```python
from build123d import *

# Parameters (mm, degrees)
F0_W           = 11
F0_H           = 30
F1_DEPTH       = 25
F1_DEPTH_BACK  = 25
F3_DEPTH       = 11
F4_R           = 10
F5_R           = 5
F6_DEPTH       = 12
F8_D           = 5
F8_START       = 11.4196012
F8_CSINK_D     = 10
F8_CSINK_ANGLE = 90


with BuildPart() as f1:
    # F0 (on Right) → F1 (new body, two sides)
    with BuildSketch(Plane.YZ) as f1_sk:
        with BuildLine():
            Line((-27.9105714739, 11), (-53.5, 11))
            Line((-53.5, 11), (-53.5, 0))
            Line((-53.5, 0), (-30, 0))
            ThreePointArc((-30, 0), (-29.4730143031, 5.5983415304), (-27.9105714739, 11))
        make_face()
        with BuildLine():
            ThreePointArc((27.9105714739, 11), (0, 30), (-27.9105714739, 11))
            ThreePointArc((-27.9105714739, 11), (-29.4730143031, 5.5983415304), (-30, 0))
            Line((-30, 0), (-19, 0))
            ThreePointArc((-19, 0), (0, 19), (19, 0))
            Line((19, 0), (30, 0))
            ThreePointArc((30, 0), (29.4730143031, 5.5983415304), (27.9105714739, 11))
        make_face()
        with BuildLine():
            Line((40, 11), (27.9105714739, 11))
            ThreePointArc((27.9105714739, 11), (29.4730143031, 5.5983415304), (30, 0))
            Line((30, 0), (51, 0))
            Line((51, 0), (51, 11))
            Line((51, 11), (40, 11))
        make_face()
        with Locations((45.5, 26)):
            Rectangle(F0_W, F0_H)
    extrude(amount=F1_DEPTH)
    extrude(f1_sk.sketch, amount=-F1_DEPTH_BACK)

    # F2 (on face) → F3 (cut)
    with BuildSketch(Plane(origin=(0, 51, 0), x_dir=(-1, 0, 0), z_dir=(0, 1, 0))):
        with BuildLine():
            Line((5, 41), (-5, 41))
            Line((-5, 41), (-5, 28.2676104225))
            ThreePointArc((-5, 28.2676104225), (0, 33.2676104225), (5, 28.2676104225))
            Line((5, 28.2676104225), (5, 41))
        make_face()
        with BuildLine():
            ThreePointArc((5, 28.2676104225), (0, 33.2676104225), (-5, 28.2676104225))
            Line((-5, 28.2676104225), (5, 28.2676104225))
        make_face()
        with BuildLine():
            Line((5, 28.2676104225), (-5, 28.2676104225))
            ThreePointArc((-5, 28.2676104225), (0, 23.2676104225), (5, 28.2676104225))
        make_face()
    extrude(amount=-F3_DEPTH, mode=Mode.SUBTRACT)

    # F4
    f4_edges = [f1.edges().sort_by_distance(p)[0] for p in [
        (25, -53.5, 5.5),
        (-25, -53.5, 5.5),
        (25, 45.5, 41),
        (-25, 45.5, 41),
    ]]
    fillet(f4_edges, radius=F4_R)

    # F5 (on face) → F6 (cut)
    with BuildSketch(Plane(origin=(0, 0, 0), x_dir=(1, 0, 0), z_dir=(0, 0, -1))):
        with Locations((-12, 43.5)):
            Circle(F5_R)
        with Locations((12, 43.5)):
            Circle(F5_R)
    extrude(amount=-F6_DEPTH, mode=Mode.SUBTRACT)

    # F8 (through all)
    # its depths count from where the whole tool has entered the part; down to there all is cleared
    with Locations(Plane.XY.offset(41).offset(-F8_START)):
        with Locations((0, 0)):
            CounterSinkHole(F8_D / 2, F8_CSINK_D / 2, counter_sink_angle=F8_CSINK_ANGLE)


solid = f1.part
```
Model file for the job. Use its own axes, mm. A direction names the side the tool comes from. Coordinates: 2 decimals unless noted, no trailing zeros. Write each loop counter-clockwise with the first axis right and the second up, starting at its lowest first coordinate (ties: lowest second). Pieces come first, ordered by that corner, then holes. Notation, with made-up numbers: (45, 31) - (95, 31) arc R30 ccw to (95, 65) - close; hole circle Ø7 at (44.25, 20.25). An arc over 180 degrees is marked (long way). Use a Markdown table: item, result. Add a question column.
Item 1: Drop flat-ended pins along their axis: pin 1 (1 mm diameter, centred on x = -19.5, z = 7, fed in from -Y); pin 2 (3 mm diameter, centred on x = -12.5, y = 5.5, fed in from +Z); pin 3 (5.5 mm diameter, centred on y = 48, z = 37, fed in from -X); pin 4 (9.5 mm diameter, centred on x = -5, y = 37, fed in from +Z). Give the stop position or say it passes through.
Item 2: Band-saw the part on B-B, the plane x = 12. Write the cut outline in (y, z), and give its area (3 significant figures).
Item 3: Two-plate mould, pull along X, no slides. Class faces 4 (the face through (0, -53.5, 6)), 5 (the face through (21.99, -50.65, 5.42)), 6 (the face through (-5, 0.11, 29.75)): pulls with the +X half, pulls with the -X half, needs draft (parallel to the pull), parting line crosses it, or undercut.
Item 4: Band-saw the part on D-D, the plane y = -37. Write the cut outline in (x, z).
Item 5: 3-axis set-ups, long thin cutter, end or side, ignore diameter. For faces 1 (the face through (0, 34, 11)), 2 (the face through (0, -41, 11)), 3 (the face through (5, -0.11, 29.75)): which of +Z, -Z, +X, -X, +Y, -Y reach the whole face in a straight line?
Item 6: Band-saw the part on A-A, the plane z = 7. Write the cut outline in (x, y).
Item 7: Drill centre lines: line 1 along X through (y, z) = (-43, 8); line 2 along Y through (x, z) = (-12, 4.75); line 3 along Y through (x, z) = (12, 5.5). Where is each one in solid material? Low to high.
Item 8: Band-saw the part on C-C, the plane x = -6. Write the cut outline in (y, z), and give its area (3 significant figures).
A:
| question | item | result |
|---|---|---|
| 1 | pin 1 | stops at y = -52.67 |
| 1 | pin 2 | stops at z = 29.73 |
| 1 | pin 3 | stops at x = -24.46 |
| 1 | pin 4 | stops at z = 41 |
| 2 | outline | (-53.5, 0) - (-48.5, 0) - (-48.5, 11) - (-53.5, 11) - close; (-38.5, 0) - (-19, 0) arc R19 cw to (19, 0) - (51, 0) - (51, 41) - (40, 41) - (40, 11) - (27.91, 11) arc R30 ccw to (-27.91, 11) - (-38.5, 11) - close |
| 2 | area | 1,570 mm² |
| 3 | face 4 | needs draft |
| 3 | face 5 | pulls with the +X half |
| 3 | face 6 | undercut |
| 4 | outline | (-25, 0) - (25, 0) - (25, 11) - (-25, 11) - close |
| 5 | face 1 | +Z, +X, -X |
| 5 | face 2 | +Z, +X, -X, -Y |
| 5 | face 3 | +Z |
| 6 | outline | (-25, -43.5) arc R10 ccw to (-15, -53.5) - (15, -53.5) arc R10 ccw to (25, -43.5) - (25, -17.66) - (-25, -17.66) - close; (-25, 17.66) - (25, 17.66) - (25, 51) - (-25, 51) - close; hole circle Ø10 at (-12, -43.5); hole circle Ø10 at (12, -43.5) |
| 7 | line 1 | x = -25 to -16.97, -7.03 to 7.03, 16.97 to 25 |
| 7 | line 2 | y = -53.5 to -48.5, -38.5 to -18.4, 18.4 to 51 |
| 7 | line 3 | y = -53.5 to -48.5, -38.5 to -18.19, 18.19 to 51 |
| 8 | outline | (-53.5, 0) - (-19, 0) arc R19 cw to (19, 0) - (51, 0) - (51, 41) - (40, 41) - (40, 11) - (27.91, 11) arc R30 ccw to (-27.91, 11) - (-53.5, 11) - close |
| 8 | area | 1,680 mm² |
